Part model, mm, in its own coordinate system. Give positions to 0.01 mm unless a question says otherwise; leave off trailing zeros. Loops run counter-clockwise (first coordinate to the right, second up) from the corner with the lowest first, then second, coordinate; pieces in that order, holes last. Notation, with made-up numbers: (-32, -37) -> (-2, -37) arc R18 ccw to (-2, -7) -> close; hole circle Ø6 at (60, -26.5). An arc over 180 degrees is marked (long way). One line per question, with ' | ' between items.
```python
from build123d import *

# Parameters (mm, degrees)
SKETCH_1_R      = 8
SKETCH_1_R_2    = 4
EXTRUDE_1_DEPTH = 5
FILLET_1_R      = 1


with BuildPart() as part:
    # 草图1 → 凸台-拉伸1 (new body, symmetric)
    with BuildSketch(Plane(origin=(0, 0, 0), x_dir=(0, 0, -1), z_dir=(1, 0, 0))):
        Circle(SKETCH_1_R)
        Circle(SKETCH_1_R_2, mode=Mode.SUBTRACT)
    extrude(amount=EXTRUDE_1_DEPTH, both=True)

    # 圆角1
    fillet_1_edges = [part.edges().sort_by_distance(p)[0] for p in [
        (-5, 0, 8),
        (5, 0, 8),
        (-5, 0, 4),
        (5, 0, 4),
    ]]
    fillet(fillet_1_edges, radius=FILLET_1_R)


solid = part.part
```
1) Drill centre lines: line 1 (Y direction, x = -1.5, z = 0); line 2 (X direction, y = -7, z = 1); line 3 (Z direction, x = 0, y = -1.75). Where is each one in solid material? Low to high.
Found:
line 1: -8 to -4, 4 to 8 | line 2: -5 to 5 | line 3: -7.81 to -3.6, 3.6 to 7.81
2) Pull direction Y, two halves, no side cores. Call faces 1 (the cylindrical face through (-0.056, -3.905, 0.867)), 2 (the flat face through (5, 5, 2)), 3 (the cylindrical face through (0.06, -7.81, 1.73)): pulls with the +Y half, pulls with the -Y half, needs draft (parallel to the pull), parting line crosses it, or undercut.
Found:
face 1: undercut | face 2: needs draft | face 3: parting line crosses it
3) Pin check, flat tips, straight feed: P1, Ø1.5, axis at x = 0.5, y = -5, coming from the -Z side; P2, Ø3, axis at x = 1, z = -4.5, coming from the +Y side; P3, Ø5, axis at x = 1, y = 4.5, coming from the -Z side. Stop position of each tip, or through.
Found:
P1: z = -6.78 | P2: y = 7.42 | P3: z = -7.75
4) Saw through at A-A (z = 0). Give the cut face in (x, y), and give its area (3 significant figures).
Found:
outline: (-5, -7) arc R1 ccw to (-4, -8) -> (4, -8) arc R1 ccw to (5, -7) -> (5, -5) arc R1 ccw to (4, -4) -> (-4, -4) arc R1 ccw to (-5, -5) -> close; (-5, 5) arc R1 ccw to (-4, 4) -> (4, 4) arc R1 ccw to (5, 5) -> (5, 7) arc R1 ccw to (4, 8) -> (-4, 8) arc R1 ccw to (-5, 7) -> close | area: 78.3 mm2
5) Saw through at C-C (x = -1.25). Give the cut face in (y, z).
Found:
outline: circle Ø16 at (0, 0); hole circle Ø8 at (0, 0)
